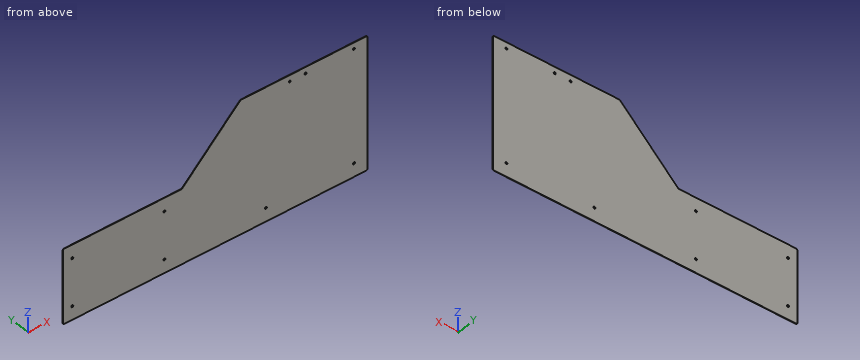
from build123d import *

# Parameters (mm, degrees)
BOSS_EXTRUDE1_DEPTH            = 1.5875
F_5_16_0_3125_DIAMETER_HOLE1_D = 7.9375
FILLET1_R                      = 6.35


with BuildPart() as part:
    # Sketch1 → Boss-Extrude1 (new body)
    with BuildSketch(Plane(origin=(0, 0, 0), x_dir=(1, 0, 0), z_dir=(0, 1, 0))):
        with BuildLine():
            Line((-1219.2, 234.95), (-745.580256121, 234.95))
            ThreePointArc((-745.580256121, 234.95), (-743.150216326, 234.466635031), (-741.090128061, 233.090128061))
            Line((-741.090128061, 233.090128061), (-509.859871939, 1.859871939))
            ThreePointArc((-509.859871939, 1.859871939), (-507.799783674, 0.483364969), (-505.369743879, 0))
            Line((-505.369743879, 0), (0, 0))
            Line((0, 0), (0, 533.4))
            Line((0, 533.4), (-1219.2, 533.4))
            Line((-1219.2, 533.4), (-1219.2, 234.95))
        make_face()
    extrude(amount=BOSS_EXTRUDE1_DEPTH)

    # 5/16 (0.3125) Diameter Hole1 (through all)
    with Locations(Plane(origin=(0, 1.5875, 0), x_dir=(1, 0, 0), z_dir=(0, 1, 0))):
        with Locations((-1181.1, 479.425), (-1181.1, 288.925), (-812.8, 288.925), (-812.8, 479.425), (-406.4, 479.425), (-53.975, 479.425), (-53.975, 25.4), (-247.65, 25.4), (-311.15, 25.4)):
            Hole(F_5_16_0_3125_DIAMETER_HOLE1_D / 2)

    # Fillet1
    fillet1_edges = [part.edges().sort_by_distance(p)[0] for p in [
        (-1219.2, 0.79375, -234.95),
        (-1219.2, 0.79375, -533.4),
        (0, 0.79375, -533.4),
        (0, 0.79375, 0),
    ]]
    fillet(fillet1_edges, radius=FILLET1_R)


solid = part.part
Geometry check sheet. Reference: the model listing, model coordinates, mm. Round coordinates to 2 decimals unless told otherwise and drop trailing zeros. Loops run counter-clockwise (first coordinate to the right, second up) from the corner with the lowest first, then second, coordinate; pieces in that order, holes last. Notation, with made-up numbers: (-32.5, -28.75) -> (-9.5, -28.75) arc R28 cw to (-9.5, -6.75) -> close; hole circle Ø4 at (40.5, -12). An arc over 180 degrees is marked (long way). Answer as a JSON object with one key per item and string values. Group by question number.
Item 1: Cross-section at C-C, the plane z = -69. Record the cut outline in (x, y), plus the area to 3 significant figures.
Item 2: Cross-section at A-A, the plane y = 0.95. Count the separate pieces of the cut face and the enclosed holes in it, plus the area to 3 significant figures.
Item 3: Cross-section at B-B, the plane x = -1031. Record the cut outline in (y, z).
Item 4: Depth check by flat-ended pin: pin 1 Ø10 at (x, z) = (-197.5, -101) entering from -Y; pin 2 Ø0.5 at (x, y) = (-923.5, 0.5) entering from +Z. Enter the tip coordinate at first touch or a pass-through.
Item 5: Thickness scan on line 1 along X through (y, z) = (0.7, -25.4); line 2 along Z through (x, y) = (-1181.1, 0.6); line 3 along Z through (x, y) = (-1155, 1.4). Record the ranges inside material, lowest first.
Determined:
{
 "1": {"outline": "(-577, 0) -> (0, 0) -> (0, 1.59) -> (-577, 1.59) -> close", "area": "916 mm²"},
 "2": {"separate pieces": "1", "enclosed holes": "9", "area": "510,000 mm²"},
 "3": {"outline": "(0, -533.4) -> (1.59, -533.4) -> (1.59, -234.95) -> (0, -234.95) -> close"},
 "4": {"pin 1": "stops at y = 0", "pin 2": "stops at z = -234.95"},
 "5": {"line 1": "x = -533.4 to -315.12, -307.18 to -251.62, -243.68 to -57.94, -50.01 to 0", "line 2": "z = -533.4 to -483.39, -475.46 to -292.89, -284.96 to -234.95", "line 3": "z = -533.4 to -234.95"}
}
